```python
from build123d import *

# Parameters (mm, degrees)
F1_DEPTH = 100
F2_R     = 10
F3_R     = 8
F4_DEPTH = 20.001


with BuildPart() as f1:
    # F0 (on Front) → F1 (new body)
    with BuildSketch(Plane.XZ):
        Polygon((0, 100), (0, 0), (70, 0), (60, 20), (20, 20), align=None)
    extrude(amount=-F1_DEPTH)

    # F2
    f2_edges = [f1.edges().sort_by_distance(p)[0] for p in [
        (60, 50, 20),
    ]]
    fillet(f2_edges, radius=F2_R)

    # F3 (on face) → F4 (cut, through all)
    with BuildSketch(Plane.XY.offset(20)):
        with Locations((35, 40)):
            Circle(F3_R)
    extrude(amount=-F4_DEPTH, mode=Mode.SUBTRACT)


solid = f1.part
```
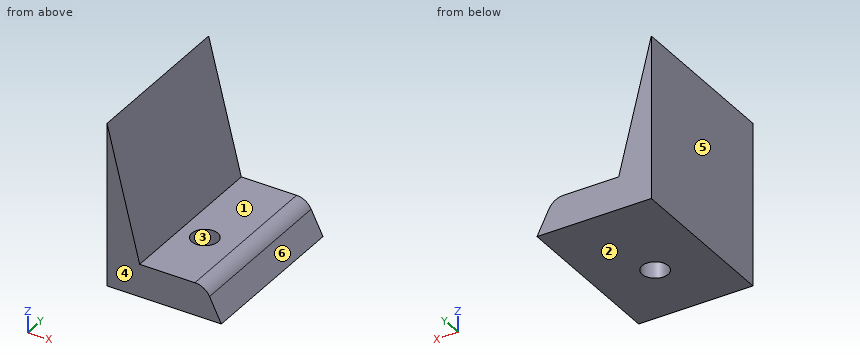
Geometry check sheet. Reference: the model listing, model coordinates, mm. Face numbers are marked on the shaded views. A direction names the side the tool comes from. Give positions to 0.01 mm unless a question says otherwise; leave off trailing zeros. Order: outer loops, then holes, each group sorted by start corner. A loop starts at its lowest first (then second) coordinate and runs counter-clockwise, first axis right, second up. Notation, with made-up numbers: (-27, 76.25) - (18, 76.25) arc R14 cw to (18, 80.25) - close; hole circle Ø6 at (23, 82). An arc over 180 degrees is marked (long way). Answer in a Markdown table with one row per item. Add a question column.
Q1. Cross-section at C-C, the plane z = 8. Enter the section's corners in (x, y).
Q2. Tool access check on the marked faces 1 and 2. Record the directions out of +Z, -Z, +X, -X, +Y, -Y that give a thin tool (end or side, any length) a straight path to the whole face; none if there is none.
Q3. Cross-section at B-B, the plane x = 35. Enter the section's corners in (y, z).
Q4. Cross-section at A-A, the plane y = 40. Enter the section's corners in (x, z).
Q5. Mould release check, pull along X, two halves, no side actions. Record for the marked faces 3, 4, 5 and 6: pulls with the +X half, pulls with the -X half, needs draft (parallel to the pull), parting line crosses it, or undercut.
Q6. Material ranges on probe 1 along Y at (x, z) = (35, 6.25); probe 2 along Z at (x, y) = (48, 41.5); probe 3 along X at (y, z) = (24, 26), recorded low to high. Write a range as from..to.
Q7. Cross-section at D-D, the plane y = 54. Enter the section's corners in (x, z), then the cut area to 3 significant figures.
Q8. Gauge pin test, flat ends, axial feed: pin 1 (1.5 mm diameter, centred on y = 43.5, z = 51, fed in from +X); pin 2 (3 mm diameter, centred on x = 42.5, y = 54, fed in from +Z); pin 3 (4 mm diameter, centred on y = 34, z = 75.5, fed in from +X) (3 decimals). Record the tip position at first contact, or that the pin passes through.
Check values:
| question | item | result |
|---|---|---|
| 1 | outline | (0, 0) - (66, 0) - (66, 100) - (0, 100) - close; hole circle Ø16 at (35, 40) |
| 2 | face 1 | +Z, +X, +Y, -Y |
| 2 | face 2 | -Z, +X, -X, +Y, -Y |
| 3 | outline | (0, 0) - (32, 0) - (32, 20) - (0, 20) - close; (48, 0) - (100, 0) - (100, 20) - (48, 20) - close |
| 4 | outline | (0, 0) - (27, 0) - (27, 20) - (20, 20) - (0, 100) - close; (43, 0) - (70, 0) - (62.76, 14.47) arc R10 ccw to (53.82, 20) - (43, 20) - close |
| 5 | face 3 | undercut |
| 5 | face 4 | needs draft |
| 5 | face 5 | pulls with the -X half |
| 5 | face 6 | pulls with the +X half |
| 6 | probe 1 | y = 0..32, 48..100 |
| 6 | probe 2 | z = 0..20 |
| 6 | probe 3 | x = 0..18.5 |
| 7 | outline | (0, 0) - (70, 0) - (62.76, 14.47) arc R10 ccw to (53.82, 20) - (20, 20) - (0, 100) - close |
| 7 | area | 2,090 mm^2 |
| 8 | pin 1 | stops at x = 12.44 |
| 8 | pin 2 | stops at z = 20 |
| 8 | pin 3 | stops at x = 6.625 |
